```python
from build123d import *

# Parameters (mm, degrees)
F0_W      = 228.6
F0_H      = 25.4
F1_DEPTH  = 25.4
F3_DEPTH  = 11.1125
F5_DEPTH  = 11.1125
F6_DEPTH  = 6.35
F8_DEPTH  = 6.35
F11_DEPTH = 25.4


with BuildPart() as f1:
    # F0 (on Front) → F1 (new body)
    with BuildSketch(Plane.XZ):
        with Locations((-4.8591513187, 4.8340088824)):
            Rectangle(F0_W, F0_H)
    extrude(amount=F1_DEPTH)

    # F2 (on face) → F3 (cut)
    with BuildSketch(Plane.XY.offset(17.5340088824)):
        Polygon((-119.1591513187, 0), (-119.1591513187, -25.4), (-106.4591513187, -12.7), (-93.7591513187, 0), align=None)
        Polygon((96.7408486813, -12.7), (109.4408486813, -25.4), (109.4408486813, 0), (84.0408486813, 0), align=None)
    extrude(amount=-F3_DEPTH, mode=Mode.SUBTRACT)

    # F4 (on face) → F5 (cut)
    with BuildSketch(Plane(origin=(0, 0, -7.8659911176), x_dir=(1, 0, 0), z_dir=(0, 0, -1))):
        Polygon((-93.7591513187, 0), (-119.1591513187, 25.4), (-119.1591513187, 0), align=None)
        Polygon((109.4408486813, 0), (109.4408486813, 25.4), (84.0408486813, 0), align=None)
    extrude(amount=-F5_DEPTH, mode=Mode.SUBTRACT)

    # F2 (on face) → F6 (cut)
    with BuildSketch(Plane.XY.offset(17.5340088824)):
        Polygon((-93.7591513187, 0), (-106.4591513187, -12.7), (96.7408486813, -12.7), (84.0408486813, 0), align=None)
    extrude(amount=-F6_DEPTH, mode=Mode.SUBTRACT)

    # F7 (on face) → F8 (cut)
    with BuildSketch(Plane.XY.offset(11.1840088824)):
        Polygon((1.4908486813, 0), (-11.2091513187, 0), (-17.5591513187, -12.7), (7.8408486813, -12.7), align=None)
    extrude(amount=-F8_DEPTH, mode=Mode.SUBTRACT)

    # F9 (on face) + F10 (on face) → F11 (cut)
    with BuildSketch(Plane.XY.offset(6.4215088824)):
        with BuildLine():
            ThreePointArc((-110.5971315457, -8.562019773), (-110.2530048029, -8.0469977067), (-110.1321635608, -7.4394877579))
            ThreePointArc((-110.1321635608, -7.4394877579), (-110.5971315457, -6.3169557427), (-111.7196635608, -5.8519877579))
            Line((-111.7196635608, -5.8519877579), (-111.7196635608, -7.4394877579))
            Line((-111.7196635608, -7.4394877579), (-110.5971315457, -8.562019773))
        make_face()
        with BuildLine():
            Line((-111.7196635608, -7.4394877579), (-111.7196635608, -5.8519877579))
            ThreePointArc((-111.7196635608, -5.8519877579), (-112.8421955759, -6.3169557427), (-113.3071635608, -7.4394877579))
            Line((-113.3071635608, -7.4394877579), (-111.7196635608, -7.4394877579))
        make_face()
        with BuildLine():
            ThreePointArc((-113.3071635608, -7.4394877579), (-112.3271735097, -8.9061465157), (-110.5971315457, -8.562019773))
            Line((-110.5971315457, -8.562019773), (-111.7196635608, -7.4394877579))
            Line((-111.7196635608, -7.4394877579), (-113.3071635608, -7.4394877579))
        make_face()
    with BuildSketch(Plane.XY.offset(6.4215088824)):
        with BuildLine():
            Line((102.0013609235, -7.4394877579), (103.5888609235, -7.4394877579))
            ThreePointArc((103.5888609235, -7.4394877579), (103.1238929386, -6.3169557427), (102.0013609235, -5.8519877579))
            Line((102.0013609235, -5.8519877579), (102.0013609235, -7.4394877579))
        make_face()
        with BuildLine():
            Line((102.0013609235, -7.4394877579), (102.0013609235, -5.8519877579))
            ThreePointArc((102.0013609235, -5.8519877579), (100.5347021656, -6.831977809), (100.8788289083, -8.562019773))
            Line((100.8788289083, -8.562019773), (102.0013609235, -7.4394877579))
        make_face()
        with BuildLine():
            ThreePointArc((100.8788289083, -8.562019773), (102.6088708723, -8.9061465157), (103.5888609235, -7.4394877579))
            Line((103.5888609235, -7.4394877579), (102.0013609235, -7.4394877579))
            Line((102.0013609235, -7.4394877579), (100.8788289083, -8.562019773))
        make_face()
    extrude(amount=-F11_DEPTH, mode=Mode.SUBTRACT)


solid = f1.part
```
Work out the finished part from the listing and answer in its coordinate system (mm). A direction names the side the tool comes from. Give positions to 0.01 mm unless a question says otherwise; leave off trailing zeros. Write each loop counter-clockwise with the first axis right and the second up, starting at its lowest first coordinate (ties: lowest second). Pieces come first, ordered by that corner, then holes.
(1) The mould has two halves that part along Y. Classify faces 4 (the flat face through (-6, 0, 2)), 5 (the flat face through (-5, -8, 4.834)), 6 (the flat face through (102, -10, 3.247)): pulls with the +Y half, pulls with the -Y half, needs draft (parallel to the pull), parting line crosses it, or undercut.
Final values:
face 4: pulls with the +Y half
face 5: undercut
face 6: needs draft
(2) Straight lines are drawn through the part: line 1 (Y direction, x = -96, z = 16.25); line 2 (Z direction, x = -71, y = -6.5); line 3 (Z direction, x = -1, y = -5.5). For each, find the intervals that lie inside material, in ascending order.
Final values:
line 1: y = -25.4 to -12.7
line 2: z = -7.87 to 11.18
line 3: z = -7.87 to 4.83
(3) Flat-ended cylindrical pins translate along their axes: pin 1 Ø10 at (x, y) = (-4, -5.5) entering from +Z; pin 2 Ø4 at (x, y) = (-48, -7) entering from +Z; pin 3 Ø2 at (x, z) = (76, 13) entering from +Y. Find the tip coordinate at first contact, or state that the pin passes through.
Final values:
pin 1: stops at z = 4.83
pin 2: stops at z = 11.18
pin 3: stops at y = -12.7
(4) The part is cut by section D-D on y = -18.75. Write down the section's boundary in (x, z), plus the area to 3 significant figures.
Final values:
outline: (-119.16, 3.25) - (-112.51, 3.25) - (-112.51, -7.87) - (102.79, -7.87) - (102.79, 3.25) - (109.44, 3.25) - (109.44, 6.42) - (102.79, 6.42) - (102.79, 17.53) - (-112.51, 17.53) - (-112.51, 6.42) - (-119.16, 6.42) - close
area: 5,510 mm2
(5) The part is cut by section C-C on y = -2. Write down the section's boundary in (x, z).
Final values:
outline: (-119.16, 3.25) - (-95.76, 3.25) - (-95.76, -7.87) - (86.04, -7.87) - (86.04, 3.25) - (109.44, 3.25) - (109.44, 6.42) - (86.04, 6.42) - (86.04, 11.18) - (2.49, 11.18) - (2.49, 4.83) - (-12.21, 4.83) - (-12.21, 11.18) - (-95.76, 11.18) - (-95.76, 6.42) - (-119.16, 6.42) - close
(6) The part is cut by section B-B on x = 65.5. Write down the section's boundary in (y, z).
Final values:
outline: (-25.4, -7.87) - (0, -7.87) - (0, 11.18) - (-12.7, 11.18) - (-12.7, 17.53) - (-25.4, 17.53) - close
(7) Which of the six approach directions +Z, -Z, +X, -X, +Y, -Y give full straight-line access (tool end or side, diameter ignored) to faces 1 (the flat face through (96.92, -12.88, -2.39)), 2 (the flat face through (99.385, -15.344, 10.821)), 3 (the flat face through (-109.46, -15.7, 10.82))?
Final values:
face 1: -Z, +X, +Y
face 2: +Z, +X, +Y
face 3: +Z, -X, +Y
(8) The part is cut by section A-A on z = 9.25. Write down the section's boundary in (x, y), plus the area to 3 significant figures.
Final values:
outline: (-119.16, -25.4) - (109.44, -25.4) - (84.04, 0) - (1.49, 0) - (7.84, -12.7) - (-17.56, -12.7) - (-11.21, 0) - (-93.76, 0) - close
area: 4,920 mm2
